from build123d import *

# Parameters (mm, degrees)
SKETCH1_W               = 9
SKETCH1_H               = 31.450000092
BOSS_EXTRUDE1_DEPTH     = 16
CUT_EXTRUDE1_DEPTH      = 35.82109913
CUT_EXTRUDE1_DEPTH_BACK = 35.82109913
SKETCH2_W               = 11
SKETCH2_H               = 31.125000096
CUT_EXTRUDE2_DEPTH      = 36.673425061
CUT_EXTRUDE2_DEPTH_BACK = 36.673425061
SKETCH3_W               = 4
SKETCH3_H               = 5
SKETCH4_W               = 11
SKETCH4_H               = 6.5
CUT_EXTRUDE3_DEPTH      = 38.434719306


with BuildPart() as part:
    # Sketch1 → Boss-Extrude1 (new body)
    with BuildSketch(Plane(origin=(0, 0, 0), x_dir=(0, 0, -1), z_dir=(1, 0, 0))):
        Polygon((-1.013717106, 26.482765172), (-2.807616659, 28.982765172), (-2.807616659, 26.482765172), align=None)
        Polygon((-2.807616659, 26.482765172), (-2.807616659, 28.982765172), (-4.057616659, 28.982765172), (-5.307616659, 23.332810224), (-5.307616659, 23.307765168), (-2.807616659, 23.307765168), align=None)
        Polygon((-11.807616659, 23.307765168), (-9.307616659, 23.307765168), (-9.307616659, 23.332810224), (-10.557616659, 28.982765172), (-11.807616659, 28.982765172), (-11.807616659, 26.482765172), align=None)
        Polygon((-13.288814039, 26.482765172), (-11.807616659, 26.482765172), (-11.807616659, 28.982765172), align=None)
        with Locations((-7.307616659, 7.582765122)):
            Rectangle(SKETCH1_W, SKETCH1_H)
    extrude(amount=-BOSS_EXTRUDE1_DEPTH)

    # Sketch2 → Cut-Extrude1 (cut, two sides: drawn at the far end of the back side and taken through both)
    with BuildSketch(Plane.XY.offset(11.807616659).offset(-CUT_EXTRUDE1_DEPTH_BACK)):
        with Locations((-8, 13.420265124)):
            Rectangle(SKETCH2_W, SKETCH2_H)
    extrude(amount=CUT_EXTRUDE1_DEPTH + CUT_EXTRUDE1_DEPTH_BACK, mode=Mode.SUBTRACT)

    # Sketch3 → Cut-Extrude2 (cut, two sides: drawn at the far end of the back side and taken through both)
    with BuildSketch(Plane(origin=(0, 0, 0), x_dir=(0, 0, -1), z_dir=(1, 0, 0)).offset(-CUT_EXTRUDE2_DEPTH_BACK)):
        with Locations((-7.307616659, 20.832810224)):
            Rectangle(SKETCH3_W, SKETCH3_H)
    extrude(amount=CUT_EXTRUDE2_DEPTH + CUT_EXTRUDE2_DEPTH_BACK, mode=Mode.SUBTRACT)

    # Sketch4 → Cut-Extrude3 (cut, through all)
    with BuildSketch(Plane(origin=(0, -2.142234924, 0), x_dir=(1, 0, 0), z_dir=(0, 1, 0))):
        with Locations((-8, -7.307616659)):
            Rectangle(SKETCH4_W, SKETCH4_H)
    extrude(amount=-CUT_EXTRUDE3_DEPTH, mode=Mode.SUBTRACT)


solid = part.part
Source: CAD feature listing. Evaluate the final solid. Frame: model axes, mm. A direction names the side the tool comes from. Give positions to 0.01 mm unless a question says otherwise; leave off trailing zeros. Write each loop counter-clockwise with the first axis right and the second up, starting at its lowest first coordinate (ties: lowest second). Pieces come first, ordered by that corner, then holes. Notation, with made-up numbers: M 7,30 L 28,30 A16 ccw 28,45 Z; hole C 6,13 d5. An arc over 180 degrees is marked long. Answer as a JSON object with one key per item and string values.
Q1. Cut plane B-B, the plane z = 6.25. Return the cut outline in (x, y), then the cut area to 3 significant figures.
Geometry check:
{"outline": "M -16,-8.14 L -13.5,-8.14 L -13.5,18.33 L -16,18.33 Z; M -2.5,-8.14 L 0,-8.14 L 0,18.33 L -2.5,18.33 Z", "area": "132 mm^2"}
Q2. Cut plane C-C, the plane z = 11.25. Return the cut outline in (x, y), then the cut area to 3 significant figures.
Geometry check:
{"outline": "M -16,-8.14 L 0,-8.14 L 0,28.98 L -2.5,28.98 L -2.5,-2.14 L -13.5,-2.14 L -13.5,28.98 L -16,28.98 Z", "area": "252 mm^2"}
Q3. Ray query, line 1 along X through (y, z) = (14, 6.5); line 2 along Z through (x, y) = (-5.5, -5.5); line 3 along Z through (x, y) = (-14.5, 21). Return the intervals inside material, ascending.
Geometry check:
{"line 1": "x = -16 to -13.5, -2.5 to 0", "line 2": "z = 2.81 to 4.06, 10.56 to 11.81", "line 3": "z = 2.81 to 5.31, 9.31 to 11.81"}
Q4. Cut plane A-A, the plane x = -7.5. Return the cut outline in (y, z).
Geometry check:
{"outline": "M -8.14,2.81 L -2.14,2.81 L -2.14,4.06 L -8.14,4.06 Z; M -8.14,10.56 L -2.14,10.56 L -2.14,11.81 L -8.14,11.81 Z"}
Q5. Access query for faces 4 (the face through (-8, -5, 4.058)), 5 (the face through (-13.5, 10, 7)), 6 (the face through (-1, 26.483, 2)), 7 (the face through (-15, 26.483, 13)), 8 (the face through (-8, -2.142, 11)). Directions: +Z, -Z, +X, -X, +Y, -Y. A direction counts if a zero-diameter tool reaches every point of the face in a straight line with its end or side. Return the directions, or none.
Geometry check:
{"face 4": "+Y, -Y", "face 5": "+Y", "face 6": "-Z, +X, -X, -Y", "face 7": "+Z, +X, -X, -Y", "face 8": "+Z, -Z, +Y"}
Q6. Mould query, pull axis X, two halves, no side actions, for faces 1 (the face through (-1, 26.483, 13)), 2 (the face through (0, 7, 7)), 3 (the face through (-8, -2.142, 3)). Classes: +X half, -X half, draft (parallel to the pull), parting line (faces both ways), or undercut.
Geometry check:
{"face 1": "draft", "face 2": "+X half", "face 3": "undercut"}
Q7. Contact query for flat-ended pins moving along their axis: P1, Ø3, axis at x = -1, y = 20, coming from the -Z side; P2, Ø1.6, axis at x = -15.5, z = 13, coming from the -Y side; P3, Ø2, axis at x = -1, z = 8, coming from the +Y side; P4, Ø6, axis at x = -12.5, z = 6, coming from the +Y side. Output: stop coordinate, or through.
Geometry check:
{"P1": "stops at z = 2.81", "P2": "stops at y = 26.48", "P3": "stops at y = 18.33", "P4": "stops at y = 28.98"}
